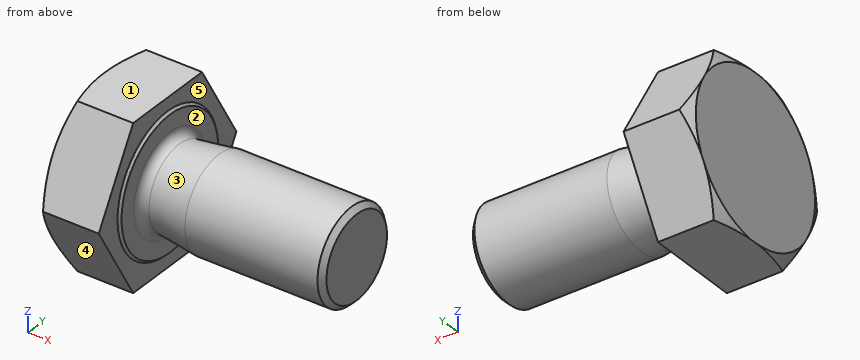
from build123d import *

# Parameters (mm, degrees)
EXTRUDE_1_DEPTH     = 2.8
SKETCH_4_R          = 7.66
SKETCH_4_R_2        = 3.5
CUT_EXTRUDE_1_DEPTH = 0.35
CUT_EXTRUDE_1_DRAFT = -60
CHAMFER_1_SIZE      = 0.222222222


with BuildPart() as part:
    # 草图3 → 凸台-拉伸1 (new body)
    with BuildSketch(Plane(origin=(0, 0, 0), x_dir=(0, 0, -1), z_dir=(1, 0, 0))):
        Polygon((3.5, 2.020725942), (0, 4.041451884), (-3.5, 2.020725942), (-3.5, -2.020725942), (0, -4.041451884), (3.5, -2.020725942), align=None)
    extrude(amount=EXTRUDE_1_DEPTH)


with BuildPart() as cut_extrude_1_tool:
    # 草图4 → 切除-拉伸1 (with draft: the straight prism first)
    with BuildSketch(Plane.ZY):
        Circle(SKETCH_4_R)
        Circle(SKETCH_4_R_2, mode=Mode.SUBTRACT)
    extrude(amount=-CUT_EXTRUDE_1_DEPTH)
    # 切除-拉伸1: the draft: its side faces are tilted about the plane it starts from
    cut_extrude_1_sides = [cut_extrude_1_tool.faces().sort_by_distance(p)[0] for p in [
        (0.175, 0, -7.66),
        (0.175, 0, -3.5),
    ]]
    draft(cut_extrude_1_sides, Plane.ZY, CUT_EXTRUDE_1_DRAFT)


with BuildPart() as part_1:
    add(part.part)

    # 切除-拉伸1: cut by cut_extrude_1_tool
    add(cut_extrude_1_tool.part, mode=Mode.SUBTRACT)

    # 草图6 → 旋转2 (revolve)
    with BuildSketch(Plane.XY, mode=Mode.PRIVATE) as revolve_2_sk:
        with BuildLine():
            Line((4.9, 2), (10.8, 2))
            Line((10.8, 2), (10.8, 0))
            Line((10.8, 0), (2.8, 0))
            Line((2.8, 0), (2.8, 2.122675))
            ThreePointArc((2.8, 2.122675), (2.919225418, 1.859534178), (3.195674814, 1.775668067))
            Line((3.195674814, 1.775668067), (4.9, 2))
        make_face()
    revolve(revolve_2_sk.sketch.rotate(Axis((2.8, 0, 0), (1, 0, 0)), 90), axis=Axis((2.8, 0, 0), (1, 0, 0)))

    # 倒角1
    chamfer_1_edges = [part_1.edges().sort_by_distance(p)[0] for p in [
        (10.8, 0, -2),
    ]]
    chamfer(chamfer_1_edges, length=CHAMFER_1_SIZE)

    # 草图8 → 切除-旋转2 (revolve, cut)
    with BuildSketch(Plane.XY, mode=Mode.PRIVATE) as cut_revolve_2_sk:
        Polygon((2.8, 2.84), (2.7, 2.94), (2.7, 7.66), (2.8, 7.66), align=None)
    revolve(cut_revolve_2_sk.sketch.rotate(Axis((0, 0, 0), (1, 0, 0)), 90), axis=Axis((0, 0, 0), (1, 0, 0)), mode=Mode.SUBTRACT)


solid = part_1.part
Source: CAD feature listing. Evaluate the final solid. Frame: model axes, mm. Face numbers are marked on the shaded views. A direction names the side the tool comes from. Coordinates: 2 decimals unless noted, no trailing zeros. Loops run counter-clockwise (first coordinate to the right, second up) from the corner with the lowest first, then second, coordinate; pieces in that order, holes last. Notation, with made-up numbers: (13.25, -2.75) - (44.25, -2.75) arc R19 cw to (44.25, 2.25) - close; hole circle Ø9 at (-32.75, 68.5). An arc over 180 degrees is marked (long way). Return JSON: item names as keys, results as strings.
Q1. Contact query for flat-ended pins moving along their axis: P1, Ø1.5, axis at x = 3, y = 3, coming from the +Z side; P2, Ø3, axis at x = 5.5, z = 1, coming from the -Y side. Output: stop coordinate, or through.
Results:
{"P1": "z = 2.99", "P2": "y = -2"}
Q2. Section A-A, the plane x = 2.25. Return loops of the section in (y, z).
Results:
{"outline": "(-4.04, 0) - (-2.02, -3.5) - (2.02, -3.5) - (4.04, 0) - (2.02, 3.5) - (-2.02, 3.5) - close"}
Q3. Mould query, pull axis X, two halves, no side actions, for the marked faces 3, 4 and 5. Classes: released by +X, released by -X, zero draft, split by the parting line, or undercut.
Results:
{"face 3": "undercut", "face 4": "zero draft", "face 5": "released by +X"}
Q4. Access query for the marked faces 1 and 2. Directions: +Z, -Z, +X, -X, +Y, -Y. A direction counts if a zero-diameter tool reaches every point of the face in a straight line with its end or side. Return the directions, or none.
Results:
{"face 1": "+Z, +X, -X, +Y, -Y", "face 2": "+X"}
Q5. Material intervals for line 1 along X through (y, z) = (1, 3.25); line 2 along X through (y, z) = (-2, 2); line 3 along Y through (x, z) = (0.75, 1), sorted ascending.
Results:
{"line 1": "0 to 2.7", "line 2": "0 to 2.8", "line 3": "-3.46 to 3.46"}
Q6. Section B-B, the plane x = 9.5. Return loops of the section in (y, z).
Results:
{"outline": "circle Ø4 at (0, 0)"}
Q7. Section C-C, the plane x = 4.75. Return loops of the section in (y, z).
Results:
{"outline": "circle Ø3.96 at (0, 0)"}
